Read the model definition and answer for the solid it produces. Units are mm, in the model's axes. A direction names the side the tool comes from. Round coordinates to 2 decimals unless told otherwise and drop trailing zeros. Order: outer loops, then holes, each group sorted by start corner. A loop starts at its lowest first (then second) coordinate and runs counter-clockwise, first axis right, second up. Notation, with made-up numbers: M 31.25,77 L 69.25,77 A11 cw 69.25,87 Z; hole C 39.5,-1 d4. An arc over 180 degrees is marked long. Answer as CSV lines item,"result".
```python
from build123d import *

# Parameters (mm, degrees)
ESQUISSE1_R        = 6.5
ESQUISSE1_R_2      = 3
BOSS_EXTRU_1_DEPTH = 5
BOSS_EXTRU_2_START = -1
ESQUISSE2_R        = 7.5
ESQUISSE2_R_2      = 3
BOSS_EXTRU_2_DEPTH = 1
CHANFREIN1_SIZE    = 0.25


with BuildPart() as part:
    # Esquisse1 → Boss.-Extru.1 (new body)
    with BuildSketch(Plane.XY):
        Circle(ESQUISSE1_R)
        Circle(ESQUISSE1_R_2, mode=Mode.SUBTRACT)
    extrude(amount=BOSS_EXTRU_1_DEPTH)

    # Esquisse2 → Boss.-Extru.2 (add)
    with BuildSketch(Plane.XY.offset(5).offset(BOSS_EXTRU_2_START)):
        Circle(ESQUISSE2_R)
        Circle(ESQUISSE2_R_2, mode=Mode.SUBTRACT)
    extrude(amount=BOSS_EXTRU_2_DEPTH)

    # Chanfrein1
    chanfrein1_edges = [part.edges().sort_by_distance(p)[0] for p in [
        (-7.5, 0, 5),
        (-6.5, 0, 0),
        (-3, 0, 5),
    ]]
    chamfer(chanfrein1_edges, length=CHANFREIN1_SIZE)


solid = part.part
```
Item 1: A cutting plane is placed at A-A, the plane x = 0. Determine the outline of the cut face in (y, z).
Ans:
outline,"M -7.5,4 L -6.5,4 L -6.5,0.25 L -6.25,0 L -3,0 L -3,4.75 L -3.25,5 L -7.25,5 L -7.5,4.75 Z; M 3,0 L 6.25,0 L 6.5,0.25 L 6.5,4 L 7.5,4 L 7.5,4.75 L 7.25,5 L 3.25,5 L 3,4.75 Z"
Item 2: Determine the mould class of faces 3 (the face through (-5.158, -3.955, 2.099)), 4 (the face through (3, 1, 0)), 5 (the face through (-3, 0, 2)) for opening direction X: +X half, -X half, draft (parallel to the pull), parting line (faces both ways), or undercut.
Ans:
face 3,"parting line"
face 4,"draft"
face 5,"undercut"
Item 3: Find the intervals of material crossed by probe 1 along Y at (x, z) = (0, 3.75); probe 2 along X at (y, z) = (2.5, 2.65); probe 3 along Z at (x, y) = (-3.25, 6), in increasing order. Write a range as [from, to].
Ans:
probe 1,"[-6.5, -3], [3, 6.5]"
probe 2,"[-6, -1.66], [1.66, 6]"
probe 3,"[4, 5]"
Item 4: A tool of negligible diameter and unlimited length cuts with its end or side. For faces 1 (the face through (-6, 3, 4)), 2 (the face through (3, -2, 5)), from which of +Z, -Z, +X, -X, +Y, -Y can it reach the whole face along a straight path? Write none if from no direction.
Ans:
face 1,"-Z"
face 2,"+Z, +X, -X, +Y, -Y"
Item 5: A cutting plane is placed at D-D, the plane z = 4.45. Determine the outline of the cut face in (x, y), and give its area (3 significant figures).
Ans:
outline,"C 0,0 d15; hole C 0,0 d6"
area,"148 mm2"
Item 6: Flat-ended cylindrical pins translate along their axes: pin 1 (1 mm diameter, centred on y = 3, z = 2, fed in from -X); pin 2 (5.5 mm diameter, centred on x = 0, y = 0, fed in from -Z); pin 3 (1.5 mm diameter, centred on x = 2.5, z = 2.5, fed in from -Y). Find the tip coordinate at first contact, or state that the pin passes through.
Ans:
pin 1,"x = -6"
pin 2,"through"
pin 3,"y = -6.26"
Item 7: A cutting plane is placed at C-C, the plane z = 1.6. Determine the outline of the cut face in (x, y), and give its area (3 significant figures).
Ans:
outline,"C 0,0 d13; hole C 0,0 d6"
area,"104 mm2"
